Design review of the part shown in the three views and the two pictorial views. Dimensions are in mm from the part's minimum x, y and z. A direction names the side the tool comes from. Round coordinates to 2 decimals unless told otherwise and drop trailing zeros. Order: outer loops, then holes, each group sorted by start corner. A loop starts at its lowest first (then second) coordinate and runs counter-clockwise, first axis right, second up. Notation, with made-up numbers: M -37.5,-24 L 17.5,-24 A18 ccw 17.5,-13 Z; hole C 87.5,-25.5 d5. An arc over 180 degrees is marked long. Write item = value, one per line. Start each with the question number.
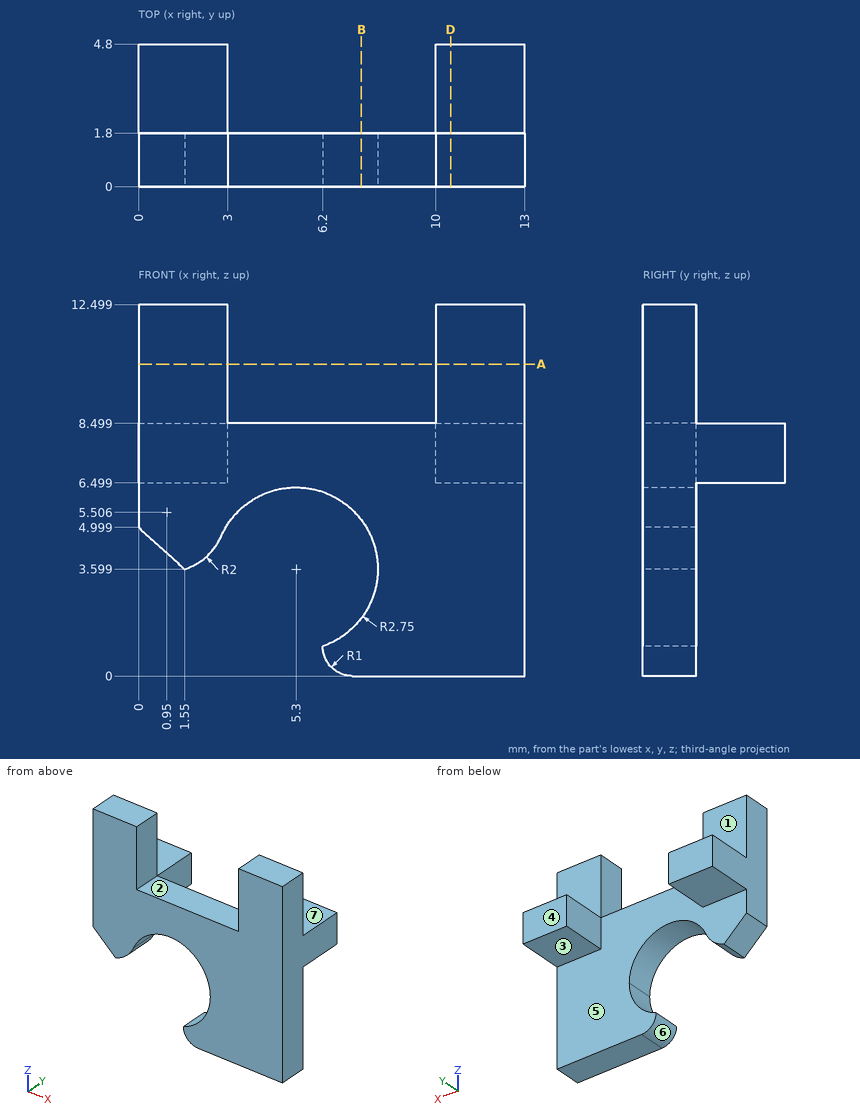
(1) Insertion check: pin 1 (2.5 mm diameter, centred on x = 1, z = 11, fed in from +Y); pin 2 (1.5 mm diameter, centred on x = 1.5, y = 3.5, fed in from -Z); pin 3 (2.5 mm diameter, centred on x = 12, y = 3.5, fed in from +Z); pin 4 (2 mm diameter, centred on y = 3, z = 3.5, fed in from -X). Each pin has a flat end and moves straight along its axis. Give the tip position at first contact, or say it passes through.
(2) We need section D-D, the plane x = 10.5. Write out the cut boundary in (y, z), then the cut area to 3 significant figures.
(3) We need section B-B, the plane x = 7.5. Write out the cut boundary in (y, z).
(4) For line 1 along X through (y, z) = (4.2, 8); line 2 along Z through (x, y) = (10.25, 2.7); line 3 along X through (y, z) = (0.55, 4.5), list the stretches that pass through material, from the lowest coordinate up.
(5) Draft analysis for pull direction X (two halves, no side actions). For the marked faces 5, 6 and 7, state which applies: released by +X, released by -X, zero draft, split by the parting line, or undercut.
(6) For the marked faces 1, 2, 3 and 4, list the 3-axis set-ups (+Z, -Z, +X, -X, +Y, -Y) from which the entire face can be reached by the end or side of a thin tool; tool diameter is ignored.
(7) We need section A-A, the plane z = 10.5. Write out the cut boundary in (x, y), then the cut area to 3 significant figures.
Values:
q1.pin_1 = 1.8
q1.pin_2 = 6.5
q1.pin_3 = 8.5
q1.pin_4 = through
q2.outline = M 0,0 L 1.8,0 L 1.8,6.5 L 4.8,6.5 L 4.8,8.5 L 1.8,8.5 L 1.8,12.5 L 0,12.5 Z
q2.area = 28.5 mm²
q3.outline = M 0,0 L 1.8,0 L 1.8,1.95 L 0,1.95 Z; M 0,5.25 L 1.8,5.25 L 1.8,8.5 L 0,8.5 Z
q4.line_1 = 0 to 3, 10 to 13
q4.line_2 = 6.5 to 8.5
q4.line_3 = 0.55 to 2.68, 7.9 to 13
q5.face_5 = undercut
q5.face_6 = released by -X
q5.face_7 = zero draft
q6.face_1 = +Z, +X, -X, +Y
q6.face_2 = +Z, +Y, -Y
q6.face_3 = -Z, +X, -X, +Y
q6.face_4 = +Z, -Z, +X, -X, +Y
q7.outline = M 0,0 L 3,0 L 3,1.8 L 0,1.8 Z; M 10,0 L 13,0 L 13,1.8 L 10,1.8 Z
q7.area = 10.8 mm²
